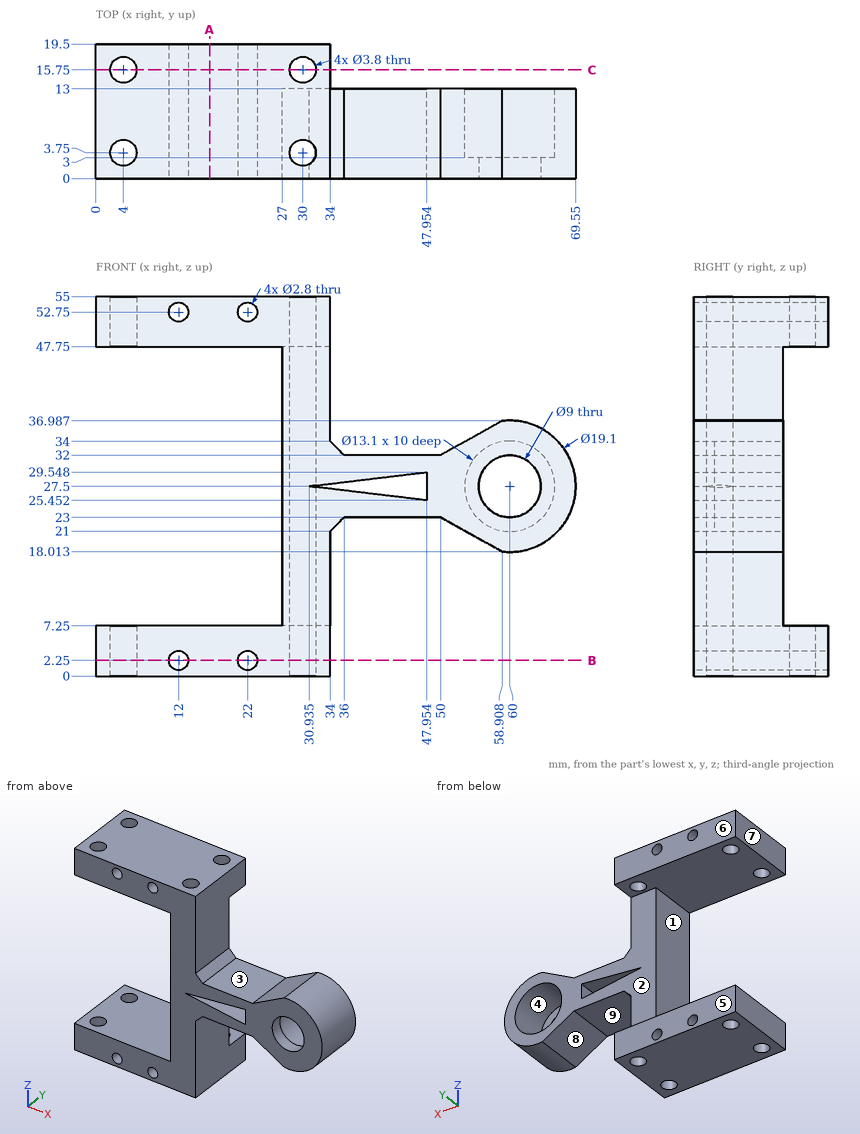
Study the drawing (mm; zero at the part's minimum x, y, z) and answer. A direction names the side the tool comes from. Give positions to 0.01 mm unless a question says otherwise; leave off trailing zeros. Loops run counter-clockwise (first coordinate to the right, second up) from the corner with the lowest first, then second, coordinate; pieces in that order, holes last. Notation, with made-up numbers: (64, 28.25) - (120, 28.25) arc R14 cw to (120, 43.25) - close; hole circle Ø4 at (-23, 73). An arc over 180 degrees is marked (long way). Return JSON: item names as keys, results as strings. Group by question number.
1. Find section A-A (x = 16.5). Write down the section's boundary in (y, z), then the cut area to 3 significant figures.
2. Find section C-C (y = 15.75). State how many separate pieces and enclosed holes the cut face has, then the cut area to 3 significant figures.
3. Which of the six approach directions +Z, -Z, +X, -X, +Y, -Y give full straight-line access (tool end or side, diameter ignored) to the marked faces 1, 2, 3, 4 and 5?
4. Straight lines are drawn through the part: line 1 (Y direction, x = 30, z = 51); line 2 (X direction, y = 9, z = 52.75); line 3 (Z direction, x = 16, y = 16.75). For each, find the intervals that lie inside material, in ascending order. Write a range as [from, to].
5. Find section B-B (z = 2.25). Write down the section's boundary in (x, y).
6. Determine the mould class of the marked faces 6, 7, 8 and 9 for opening direction X: pulls with the +X half, pulls with the -X half, needs draft (parallel to the pull), parting line crosses it, or undercut.
7. Given pin 1 Ø5 at (y, z) = (4, 21) entering from -X; pin 2 Ø10.5 at (x, z) = (57, 29.5) entering from +Y; pin 3 Ø10.5 at (x, y) = (39.5, 4.5) entering from -Z, each flat-ended and moving along its own axis, determine where each tip first touches the part or whether it passes through.
Verdict:
{
 "1": {"outline": "(0, 0) - (19.5, 0) - (19.5, 7.25) - (0, 7.25) - close; (0, 47.75) - (19.5, 47.75) - (19.5, 55) - (0, 55) - close", "area": "283 mm^2"},
 "2": {"separate pieces": "6", "enclosed holes": "4", "area": "358 mm^2"},
 "3": {"face 1": "-X, +Y, -Y", "face 2": "+X, -X, +Y", "face 3": "+Z, +Y, -Y", "face 4": "+Y", "face 5": "+Z, -Z, +X, -X, +Y"},
 "4": {"line 1": "y = [0, 1.85], [5.65, 13.85], [17.65, 19.5]", "line 2": "x = [0, 10.6], [13.4, 20.6], [23.4, 34]", "line 3": "z = [0, 7.25], [47.75, 55]"},
 "5": {"outline": "(0, 0) - (10.6, 0) - (10.6, 19.5) - (0, 19.5) - close; (13.4, 0) - (20.6, 0) - (20.6, 19.5) - (13.4, 19.5) - close; (23.4, 0) - (34, 0) - (34, 19.5) - (23.4, 19.5) - close; hole circle Ø3.8 at (4, 3.75); hole circle Ø3.8 at (4, 15.75); hole circle Ø3.8 at (30, 3.75); hole circle Ø3.8 at (30, 15.75)"},
 "6": {"face 6": "needs draft", "face 7": "pulls with the -X half", "face 8": "undercut", "face 9": "undercut"},
 "7": {"pin 1": "stops at x = 27", "pin 2": "stops at y = 13", "pin 3": "stops at z = 21.25"}
}
